from build123d import *

# Parameters (mm, degrees)
SKETCH1_R           = 6
BOSS_EXTRUDE1_DEPTH = 2.5


with BuildPart() as part:
    # Sketch1 → Boss-Extrude1 (new, symmetric)
    with BuildSketch(Plane(origin=(0, 0, 0), x_dir=(0, 1, 0), z_dir=(0, 0, 1))):
        with BuildLine():
            Line((0, 11), (205, 11))
            Line((205, 11), (205, 5))
            Line((205, 5), (200, 5))
            Line((200, 5), (200, -5))
            Line((200, -5), (205, -5))
            Line((205, -5), (205, -11))
            Line((205, -11), (0, -11))
            ThreePointArc((0, -11), (-11, 0), (0, 11))
        make_face()
        with Locations(Location((0, 0, 0), (0, 0, 270))):
            Circle(SKETCH1_R, mode=Mode.SUBTRACT)
    extrude(amount=BOSS_EXTRUDE1_DEPTH, both=True)


solid = part.part
The listing builds one solid part. Answer for the finished solid, in the listing's coordinates (mm). A direction names the side the tool comes from. Coordinates: 2 decimals unless noted, no trailing zeros. Write each loop counter-clockwise with the first axis right and the second up, starting at its lowest first coordinate (ties: lowest second). Pieces come first, ordered by that corner, then holes. Notation, with made-up numbers: (-38, 46) - (-4, 46) arc R33 ccw to (-4, 79) - close; hole circle Ø1 at (8, 45). An arc over 180 degrees is marked (long way). Answer as CSV lines item,"result".
1. Determine the mould class of faces 3 (the cylindrical face through (0, -11, 0)), 4 (the cylindrical face through (5.723, 1.802, -0.035)), 5 (the flat face through (0, 200, 0)), 6 (the flat face through (11, 104, 0)) for opening direction X: +X half, -X half, draft (parallel to the pull), parting line (faces both ways), or undercut.
Computed values:
face 3,"parting line"
face 4,"undercut"
face 5,"undercut"
face 6,"+X half"
2. A tool of negligible diameter and unlimited length cuts with its end or side. For faces 1 (the flat face through (5, 202, 0)), 2 (the flat face through (-11, 101, 0)), from which of +Z, -Z, +X, -X, +Y, -Y can it reach the whole face along a straight path? Write none if from no direction.
Computed values:
face 1,"+Z, -Z, +Y"
face 2,"+Z, -Z, -X, +Y, -Y"
3. Given P1, Ø1.5, axis at x = -2.5, z = -0.5, coming from the +Y side; P2, Ø1, axis at x = 5.5, z = 0.5, coming from the -Y side, each flat-ended and moving along its own axis, determine where each tip first touches the part or whether it passes through.
Computed values:
P1,"stops at y = 200"
P2,"stops at y = -9.8"
4. Straight lines are drawn through the part: line 1 (Y direction, x = 0, z = -1.15); line 2 (Y direction, x = 2.25, z = 2.1); line 3 (Y direction, x = -7.25, z = -1.85). For each, find the intervals that lie inside material, in ascending order. Write a range as [from, to].
Computed values:
line 1,"y = [-11, -6], [6, 200]"
line 2,"y = [-10.77, -5.56], [5.56, 200]"
line 3,"y = [-8.27, 205]"
5. Find section A-A (x = 0). Give the vertices of the cut face in (y, z), plus the area to 3 significant figures.
Computed values:
outline,"(-11, -2.5) - (-6, -2.5) - (-6, 2.5) - (-11, 2.5) - close; (6, -2.5) - (200, -2.5) - (200, 2.5) - (6, 2.5) - close"
area,"995 mm²"
6. Find section B-B (z = 0.25). Give the vertices of the cut face in (x, y), plus the area to 3 significant figures.
Computed values:
outline,"(-11, 0) arc R11 ccw to (11, 0) - (11, 205) - (5, 205) - (5, 200) - (-5, 200) - (-5, 205) - (-11, 205) - close; hole circle Ø12 at (0, 0)"
area,"4,540 mm²"
